```python
from build123d import *

# Parameters (mm, degrees)
F0_R         = 4.8298181264
F1_DEPTH     = 25
F2_DEPTH     = 10
F3_R         = 2
F4_R         = 1.5870534729
F5_DEPTH     = 0.5
F6_R         = 2.6450892659
F7_DEPTH     = 41.5
F8_R         = 1.6875975258
F9_DEPTH     = 47.4
F10_S7_R     = 1.6875975258
F10_T8_DEPTH = 5
F11_R        = 3.2484404645
F12_DEPTH    = 41.4
F13_SIZE     = 1
F14_R        = 1.2894560282
F15_DEPTH    = 48.4
F16_SIZE     = 1


# Not quite as in the source:
# - a fillet or chamfer that OpenCascade refuses, or shapes differently, is made with other operations: its cross-section is extruded or revolved along the edge and cut away or added


with BuildPart() as f1:
    # F0 (on Front) → F1 (new body)
    with BuildSketch(Plane.XZ):
        Circle(F0_R)
    extrude(amount=F1_DEPTH)

    # F2 (add): a face of the model
    f2_faces = [f1.faces().sort_by_distance(p)[0] for p in [
        (0, -25, 0),
    ]]
    extrude(f2_faces, amount=F2_DEPTH)

    # F3
    f3_edges = [f1.edges().sort_by_distance(p)[0] for p in [
        (-4.829818, -35, 0),
    ]]
    fillet(f3_edges, radius=F3_R)

    # F4 (on Front) → F5 (cut)
    with BuildSketch(Plane.XZ):
        Circle(F4_R)
    extrude(amount=F5_DEPTH, mode=Mode.SUBTRACT)

    # F6 (on Front) → F7 (join)
    with BuildSketch(Plane.XZ):
        Circle(F6_R)
    extrude(amount=F7_DEPTH)

    # F8 (on Front) → F9 (join)
    with BuildSketch(Plane.XZ):
        Circle(F8_R)
    extrude(amount=F9_DEPTH)

    # F10: chamfer of 1 on 2 edges, made by hand

    # F10_s1 → F10_t2 (revolve, cut)
    with BuildSketch(Plane.XY):
        Polygon((1.6875975258, -46.4), (0.6875975258, -47.4), (1.6875975258, -47.4), align=None)
    revolve(axis=Axis((0, -47.4, 0), (0, -1, 0)), mode=Mode.SUBTRACT)


with BuildPart() as f10_tool4:
    # F10_s5 → F10_t6 (revolve)
    with BuildSketch(Plane.XY):
        Polygon((2.6450892659, -40.5), (1.6450892659, -41.5), (2.6450892659, -41.5), align=None)
    revolve(axis=Axis((0, -41.5, 0), (0, -1, 0)))

    # F10_s7 → F10_t8 (cut, symmetric)
    with BuildSketch(Plane.XZ.offset(41)):
        Circle(F10_S7_R)
    extrude(amount=F10_T8_DEPTH, both=True, mode=Mode.SUBTRACT)


with BuildPart() as f1_1:
    add(f1.part)

    # F10_t3: cut F10_tool4
    add(f10_tool4.part, mode=Mode.SUBTRACT)

    # F11 (on Front) → F12 (join)
    with BuildSketch(Plane.XZ):
        Circle(F11_R)
    extrude(amount=F12_DEPTH)

    # F13
    f13_edges = [f1_1.edges().sort_by_distance(p)[0] for p in [
        (-3.24844, -41.4, 0),
    ]]
    chamfer(f13_edges, length=F13_SIZE)

    # F14 (on Front) → F15 (join)
    with BuildSketch(Plane.XZ):
        Circle(F14_R)
    extrude(amount=F15_DEPTH)

    # F16
    f16_edges = [f1_1.edges().sort_by_distance(p)[0] for p in [
        (-1.289456, -48.4, 0),
    ]]
    chamfer(f16_edges, length=F16_SIZE)


solid = f1_1.part
```
Geometry: final body of the model. Coordinates: model frame, mm. A direction names the side the tool comes from. Coordinates: 2 decimals unless noted, no trailing zeros. Loops run counter-clockwise (first coordinate to the right, second up) from the corner with the lowest first, then second, coordinate; pieces in that order, holes last. Notation, with made-up numbers: (-22, -19) -> (23, -19) arc R15 ccw to (23, 9) -> close; hole circle Ø11 at (63.25, -8). An arc over 180 degrees is marked (long way). Use a Markdown table: item, result. Add a question column.
(1) Pin query (flat end, axial travel): pin 1 Ø3.5 at (x, z) = (-0.5, 0) entering from -Y. Return the tip coordinate at first contact, or that it passes through.
(2) Section query B-B, the plane y = -37. Return loops of the section in (x, z), plus the area to 3 significant figures.
(3) Section query A-A, the plane y = -4. Return loops of the section in (x, z).
(4) Access query for faces 1 (the cylindrical face through (-0.28, -47.09, -1.26)), 2 (the cylindrical face through (-3.83, -16.27, -2.94)). Directions: +Z, -Z, +X, -X, +Y, -Y. A direction counts if a zero-diameter tool reaches every point of the face in a straight line with its end or side. Return the directions, or none.
(5) Line query: line 1 along Y through (x, z) = (1.5, -1.5); line 2 along Z through (x, y) = (0, -38); line 3 along Y through (x, z) = (0, 1). Output: solid intervals per line, ascending.
Answer:
| question | item | result |
|---|---|---|
| 1 | pin 1 | stops at y = -48.4 |
| 2 | outline | circle Ø6.5 at (0, 0) |
| 2 | area | 33.2 mm^2 |
| 3 | outline | circle Ø9.66 at (0, 0) |
| 4 | face 1 | -Y |
| 4 | face 2 | +Y, -Y |
| 5 | line 1 | y = -41.4 to 0 |
| 5 | line 2 | z = -3.25 to 3.25 |
| 5 | line 3 | y = -47.69 to 0 |
